Geometry check sheet. Reference: the model listing, model coordinates, mm. A direction names the side the tool comes from. Coordinates: 2 decimals unless noted, no trailing zeros. Order: outer loops, then holes, each group sorted by start corner. A loop starts at its lowest first (then second) coordinate and runs counter-clockwise, first axis right, second up. Notation, with made-up numbers: (17.25, 22.5) - (47.25, 22.5) arc R13 cw to (47.25, 40.5) - close; hole circle Ø2 at (-6.75, 11.25). An arc over 180 degrees is marked (long way). Use CSV: the item, a comma, the result in double quotes. Start each with the question number.
1) Draft check along X on faces 1 (the flat face through (-584.729, -219, 335)), 2 (the flat face through (-288, -425.45, 121)). Enter one of: released by +X, released by -X, zero draft, split by the parting line, or undercut.
2) Depth check by flat-ended pin: P1, Ø2, axis at x = -641.5, y = -275.5, coming from the +Z side; P2, Ø8, axis at x = -628.5, z = -284.5, coming from the -Y side. Enter the tip coordinate at first touch or a pass-through.
3) Sectioned sample at C-C, the plane y = -87.5. Count the separate pieces of the cut face and the enclosed holes in it, and give its area (3 significant figures).
4) Sectioned sample at A-A, the plane z = 363. Record the cut outline in (x, y), and give its area (3 significant figures).
5) Thickness scan on probe 1 along X at (y, z) = (-288.5, 4); probe 2 along X at (y, z) = (-310.5, 1177); probe 3 along Y at (x, z) = (-629.5, 348.5). Record the ranges inside material, lowest first. Write a range as [from, to].
6) Tool access check on faces 3 (the flat face through (324.909, -219, 1259)), 4 (the flat face through (-128, -219, 832.363)). Record the directions out of +Z, -Z, +X, -X, +Y, -Y that give a thin tool (end or side, any length) a straight path to the whole face; none if there is none.
from build123d import *

# Parameters (mm, degrees)
F0_W     = 1257.3
F0_H     = 2165.35
F1_DEPTH = 19.05
F2_W     = 19.05
F2_H     = 304.8
F2_W_2   = 290.5125
F2_H_2   = 19.05
F3_DEPTH = 406.4


with BuildPart() as f1:
    # F0 (on Front) → F1 (new body)
    with BuildSketch(Plane.XZ):
        with Locations((-284.6911793649, 276.7382148782)):
            Rectangle(F0_W, F0_H)
    extrude(amount=F1_DEPTH)

    # F2 (on face) → F3 (join)
    with BuildSketch(Plane.XZ.offset(19.05)):
        Polygon((-913.3411793649, 1359.4132148782), (-913.3411793649, -805.9367851218), (-894.2911793649, -805.9367851218), (-894.2911793649, -786.8867851218), (-894.2911793649, -482.0867851218), (-894.2911793649, -463.0367851218), (-894.2911793649, -158.2367851218), (-894.2911793649, -139.1867851218), (-894.2911793649, 165.6132148782), (-894.2911793649, 184.6632148782), (-894.2911793649, 489.4632148782), (-894.2911793649, 508.5132148782), (-894.2911793649, 813.3132148782), (-894.2911793649, 832.3632148782), (-894.2911793649, 1137.1632148782), (-894.2911793649, 1156.2132148782), (-894.2911793649, 1359.4132148782), align=None)
        Polygon((-894.2911793649, -786.8867851218), (-894.2911793649, -805.9367851218), (324.9088206351, -805.9367851218), (324.9088206351, -786.8867851218), (34.3963206351, -786.8867851218), (19.05, -786.8867851218), (15.3463206351, -786.8867851218), (0, -786.8867851218), (-275.1661793649, -786.8867851218), (-294.2161793649, -786.8867851218), (-584.7286793649, -786.8867851218), (-603.7786793649, -786.8867851218), align=None)
        Polygon((324.9088206351, -786.8867851218), (324.9088206351, -805.9367851218), (343.9588206351, -805.9367851218), (343.9588206351, 1359.4132148782), (324.9088206351, 1359.4132148782), (324.9088206351, 1156.2132148782), (324.9088206351, 1137.1632148782), (324.9088206351, 832.3632148782), (324.9088206351, 813.3132148782), (324.9088206351, 508.5132148782), (324.9088206351, 489.4632148782), (324.9088206351, 184.6632148782), (324.9088206351, 165.6132148782), (324.9088206351, -139.1867851218), (324.9088206351, -158.2367851218), (324.9088206351, -463.0367851218), (324.9088206351, -482.0867851218), align=None)
        Polygon((324.9088206351, 1156.2132148782), (-894.2911793649, 1156.2132148782), (-894.2911793649, 1137.1632148782), (-603.7786793649, 1137.1632148782), (-584.7286793649, 1137.1632148782), (-294.2161793649, 1137.1632148782), (-275.1661793649, 1137.1632148782), (0, 1137.1632148782), (15.3463206351, 1137.1632148782), (19.05, 1137.1632148782), (34.3963206351, 1137.1632148782), (324.9088206351, 1137.1632148782), align=None)
        with Locations((-594.2536793649, 660.9132148782)):
            Rectangle(F2_W, F2_H)
        with Locations((-594.2536793649, 984.7632148782)):
            Rectangle(F2_W, F2_H)
        with Locations((-749.0349293649, 822.8382148782)):
            Rectangle(F2_W_2, F2_H_2)
        with Locations((-439.4724293649, 822.8382148782)):
            Rectangle(F2_W_2, F2_H_2)
        with Locations((-594.2536793649, 822.8382148782)):
            Rectangle(F2_W, F2_H_2)
        with Locations((-284.6911793649, 822.8382148782)):
            Rectangle(F2_W, F2_H_2)
        with Locations((-129.9099293649, 822.8382148782)):
            Rectangle(F2_W_2, F2_H_2)
        with Locations((24.8713206351, 822.8382148782)):
            Rectangle(F2_W, F2_H_2)
        with Locations((179.6525706351, 822.8382148782)):
            Rectangle(F2_W_2, F2_H_2)
        Polygon((34.3963206351, 832.3632148782), (34.3963206351, 1137.1632148782), (19.05, 1137.1632148782), (15.3463206351, 1137.1632148782), (15.3463206351, 832.3632148782), align=None)
        with Locations((-284.6911793649, 984.7632148782)):
            Rectangle(F2_W, F2_H)
        with Locations((-284.6911793649, 660.9132148782)):
            Rectangle(F2_W, F2_H)
        with Locations((24.8713206351, 660.9132148782)):
            Rectangle(F2_W, F2_H)
        with Locations((-749.0349293649, 498.9882148782)):
            Rectangle(F2_W_2, F2_H_2)
        with Locations((-594.2536793649, 498.9882148782)):
            Rectangle(F2_W, F2_H_2)
        with Locations((-439.4724293649, 498.9882148782)):
            Rectangle(F2_W_2, F2_H_2)
        with Locations((-284.6911793649, 498.9882148782)):
            Rectangle(F2_W, F2_H_2)
        with Locations((-129.9099293649, 498.9882148782)):
            Rectangle(F2_W_2, F2_H_2)
        with Locations((24.8713206351, 498.9882148782)):
            Rectangle(F2_W, F2_H_2)
        with Locations((179.6525706351, 498.9882148782)):
            Rectangle(F2_W_2, F2_H_2)
        with Locations((-749.0349293649, 175.1382148782)):
            Rectangle(F2_W_2, F2_H_2)
        with Locations((-594.2536793649, 175.1382148782)):
            Rectangle(F2_W, F2_H_2)
        with Locations((-439.4724293649, 175.1382148782)):
            Rectangle(F2_W_2, F2_H_2)
        with Locations((-284.6911793649, 175.1382148782)):
            Rectangle(F2_W, F2_H_2)
        with Locations((-129.9099293649, 175.1382148782)):
            Rectangle(F2_W_2, F2_H_2)
        with Locations((24.8713206351, 175.1382148782)):
            Rectangle(F2_W, F2_H_2)
        with Locations((179.6525706351, 175.1382148782)):
            Rectangle(F2_W_2, F2_H_2)
        with Locations((24.8713206351, 337.0632148782)):
            Rectangle(F2_W, F2_H)
        with Locations((-284.6911793649, 337.0632148782)):
            Rectangle(F2_W, F2_H)
        with Locations((-594.2536793649, 337.0632148782)):
            Rectangle(F2_W, F2_H)
        with Locations((-749.0349293649, -148.7117851218)):
            Rectangle(F2_W_2, F2_H_2)
        with Locations((-594.2536793649, -148.7117851218)):
            Rectangle(F2_W, F2_H_2)
        with Locations((-439.4724293649, -148.7117851218)):
            Rectangle(F2_W_2, F2_H_2)
        with Locations((-284.6911793649, -148.7117851218)):
            Rectangle(F2_W, F2_H_2)
        with Locations((-129.9099293649, -148.7117851218)):
            Rectangle(F2_W_2, F2_H_2)
        with Locations((24.8713206351, -148.7117851218)):
            Rectangle(F2_W, F2_H_2)
        with Locations((179.6525706351, -148.7117851218)):
            Rectangle(F2_W_2, F2_H_2)
        with Locations((-594.2536793649, 13.2132148782)):
            Rectangle(F2_W, F2_H)
        with Locations((-284.6911793649, 13.2132148782)):
            Rectangle(F2_W, F2_H)
        with Locations((24.8713206351, 13.2132148782)):
            Rectangle(F2_W, F2_H)
        with Locations((-749.0349293649, -472.5617851218)):
            Rectangle(F2_W_2, F2_H_2)
        with Locations((-594.2536793649, -472.5617851218)):
            Rectangle(F2_W, F2_H_2)
        with Locations((-439.4724293649, -472.5617851218)):
            Rectangle(F2_W_2, F2_H_2)
        with Locations((-284.6911793649, -472.5617851218)):
            Rectangle(F2_W, F2_H_2)
        with Locations((-129.9099293649, -472.5617851218)):
            Rectangle(F2_W_2, F2_H_2)
        with Locations((24.8713206351, -472.5617851218)):
            Rectangle(F2_W, F2_H_2)
        with Locations((179.6525706351, -472.5617851218)):
            Rectangle(F2_W_2, F2_H_2)
        with Locations((-594.2536793649, -310.6367851218)):
            Rectangle(F2_W, F2_H)
        with Locations((-284.6911793649, -310.6367851218)):
            Rectangle(F2_W, F2_H)
        with Locations((24.8713206351, -310.6367851218)):
            Rectangle(F2_W, F2_H)
        Polygon((19.05, -786.8867851218), (34.3963206351, -786.8867851218), (34.3963206351, -482.0867851218), (15.3463206351, -482.0867851218), (15.3463206351, -786.8867851218), align=None)
        with Locations((-284.6911793649, -634.4867851218)):
            Rectangle(F2_W, F2_H)
        with Locations((-594.2536793649, -634.4867851218)):
            Rectangle(F2_W, F2_H)
    extrude(amount=F3_DEPTH)


solid = f1.part
Evaluation:
1,face 1,"undercut"
1,face 2,"zero draft"
2,P1,"z = 1156.21"
2,P2,"y = -19.05"
3,separate pieces,"1"
3,enclosed holes,"24"
3,area,"350,000 mm²"
4,outline,"(-913.34, -425.45) - (-894.29, -425.45) - (-894.29, -19.05) - (-603.78, -19.05) - (-603.78, -425.45) - (-584.73, -425.45) - (-584.73, -19.05) - (-294.22, -19.05) - (-294.22, -425.45) - (-275.17, -425.45) - (-275.17, -19.05) - (15.35, -19.05) - (15.35, -425.45) - (34.4, -425.45) - (34.4, -19.05) - (324.91, -19.05) - (324.91, -425.45) - (343.96, -425.45) - (343.96, 0) - (-913.34, 0) - close"
4,area,"62,700 mm²"
5,probe 1,"[-913.34, -894.29], [-603.78, -584.73], [-294.22, -275.17], [15.35, 34.4], [324.91, 343.96]"
5,probe 2,"[-913.34, -894.29], [324.91, 343.96]"
5,probe 3,"[-19.05, 0]"
6,face 3,"+Z, -Y"
6,face 4,"-Y"
